Build history of the part. All positions in model axes, mm. A direction names the side the tool comes from. Coordinates: 2 decimals unless noted, no trailing zeros. Write each loop counter-clockwise with the first axis right and the second up, starting at its lowest first coordinate (ties: lowest second). Pieces come first, ordered by that corner, then holes.
```python
from build123d import *

# Parameters (mm, degrees)
SKETCH_1_W      = 188
SKETCH_1_H      = 75
SKETCH_1_W_2    = 60
SKETCH_1_H_2    = 45
SKETCH_1_R      = 1.5
SKETCH_1_W_3    = 80
SKETCH_1_H_3    = 55
EXTRUDE_1_DEPTH = 4
FILLET_1_R      = 3


with BuildPart() as part:
    # 草图1 → 凸台-拉伸1 (new body)
    with BuildSketch(Plane(origin=(0, 0, 0), x_dir=(1, 0, 0), z_dir=(0, 1, 0))):
        with Locations((31.5, 0)):
            Rectangle(SKETCH_1_W, SKETCH_1_H)
        with Locations((82.5, 0)):
            Rectangle(SKETCH_1_W_2, SKETCH_1_H_2, mode=Mode.SUBTRACT)
        with Locations(Location((-58.4, -33, 0), (0, 0, 270))):
            Circle(SKETCH_1_R, mode=Mode.SUBTRACT)
        with Locations(Location((56.4, -33, 0), (0, 0, 270))):
            Circle(SKETCH_1_R, mode=Mode.SUBTRACT)
        with Locations(Location((46.5, -23.5, 0), (0, 0, 270))):
            Circle(SKETCH_1_R, mode=Mode.SUBTRACT)
        with Locations((-2.5, 0)):
            Rectangle(SKETCH_1_W_3, SKETCH_1_H_3, mode=Mode.SUBTRACT)
        with Locations(Location((-53.5, 26.5, 0), (0, 0, 270))):
            Circle(SKETCH_1_R, mode=Mode.SUBTRACT)
        with Locations(Location((-58.4, 33, 0), (0, 0, 270))):
            Circle(SKETCH_1_R, mode=Mode.SUBTRACT)
        with Locations(Location((46.5, 26.5, 0), (0, 0, 270))):
            Circle(SKETCH_1_R, mode=Mode.SUBTRACT)
        with Locations(Location((56.4, 33, 0), (0, 0, 270))):
            Circle(SKETCH_1_R, mode=Mode.SUBTRACT)
        with Locations(Location((66.5, 32, 0), (0, 0, 270))):
            Circle(SKETCH_1_R, mode=Mode.SUBTRACT)
        with Locations(Location((118.5, 32, 0), (0, 0, 270))):
            Circle(SKETCH_1_R, mode=Mode.SUBTRACT)
        with Locations(Location((66.5, -32, 0), (0, 0, 270))):
            Circle(SKETCH_1_R, mode=Mode.SUBTRACT)
        with Locations(Location((118.5, -32, 0), (0, 0, 270))):
            Circle(SKETCH_1_R, mode=Mode.SUBTRACT)
        with Locations(Location((118.5, -23.5, 0), (0, 0, 270))):
            Circle(SKETCH_1_R, mode=Mode.SUBTRACT)
        with Locations(Location((118.5, 18.5, 0), (0, 0, 270))):
            Circle(SKETCH_1_R, mode=Mode.SUBTRACT)
    extrude(amount=EXTRUDE_1_DEPTH)

    # 圆角1
    fillet_1_edges = [part.edges().sort_by_distance(p)[0] for p in [
        (52.5, 2, 22.5),
        (112.5, 2, 22.5),
        (112.5, 2, -22.5),
        (52.5, 2, -22.5),
        (-42.5, 2, 27.5),
        (37.5, 2, 27.5),
        (37.5, 2, -27.5),
        (-42.5, 2, -27.5),
        (125.5, 2, 37.5),
        (-62.5, 2, 37.5),
        (-62.5, 2, -37.5),
        (125.5, 2, -37.5),
    ]]
    fillet(fillet_1_edges, radius=FILLET_1_R)


solid = part.part
```
1. Saw through at B-B on z = -8. List the corners of the cut face in (x, y), plus the area to 3 significant figures.
Computed values:
outline: (-62.5, 0) - (-42.5, 0) - (-42.5, 4) - (-62.5, 4) - close; (37.5, 0) - (52.5, 0) - (52.5, 4) - (37.5, 4) - close; (112.5, 0) - (125.5, 0) - (125.5, 4) - (112.5, 4) - close
area: 192 mm2
2. Saw through at C-C on x = -14.5. List the corners of the cut face in (y, z), plus the area to 3 significant figures.
Computed values:
outline: (0, -37.5) - (4, -37.5) - (4, -27.5) - (0, -27.5) - close; (0, 27.5) - (4, 27.5) - (4, 37.5) - (0, 37.5) - close
area: 80.0 mm2
3. Saw through at D-D on y = 1.05. State how many separate pieces and enclosed holes the cut face has, plus the area to 3 significant figures.
Computed values:
separate pieces: 1
enclosed holes: 15
area: 6,920 mm2
4. Mould opens along Z. For faces 1 (the face through (30, 2, -37.5)), 2 (the face through (-42.5, 2, 0)), 3 (the face through (-62.5, 2, 0)) say: +Z half, -Z half, draft (parallel to the pull), parting line (faces both ways), or undercut.
Computed values:
face 1: -Z half
face 2: undercut
face 3: draft
5. 3-axis set-ups, long thin cutter, end or side, ignore diameter. For faces 4 (the face through (-3, 2, -27.5)), 5 (the face through (30, 2, 37.5)): which of +Z, -Z, +X, -X, +Y, -Y reach the whole face in a straight line?
Computed values:
face 4: +Y, -Y
face 5: +Z, +X, -X, +Y, -Y
6. Probe line 1 along X through (y, z) = (3.75, -4.5); line 2 along X through (y, z) = (3.15, -18.5); line 3 along X through (y, z) = (3.5, -23). List the from-to ranges inside material, lowest first.
Computed values:
line 1: x = -62.5 to -42.5, 37.5 to 52.5, 112.5 to 125.5
line 2: x = -62.5 to -42.5, 37.5 to 52.5, 112.5 to 117, 120 to 125.5
line 3: x = -62.5 to -42.5, 37.5 to 125.5
7. Saw through at A-A on x = 100. List the corners of the cut face in (y, z).
Computed values:
outline: (0, -37.5) - (4, -37.5) - (4, -22.5) - (0, -22.5) - close; (0, 22.5) - (4, 22.5) - (4, 37.5) - (0, 37.5) - close
